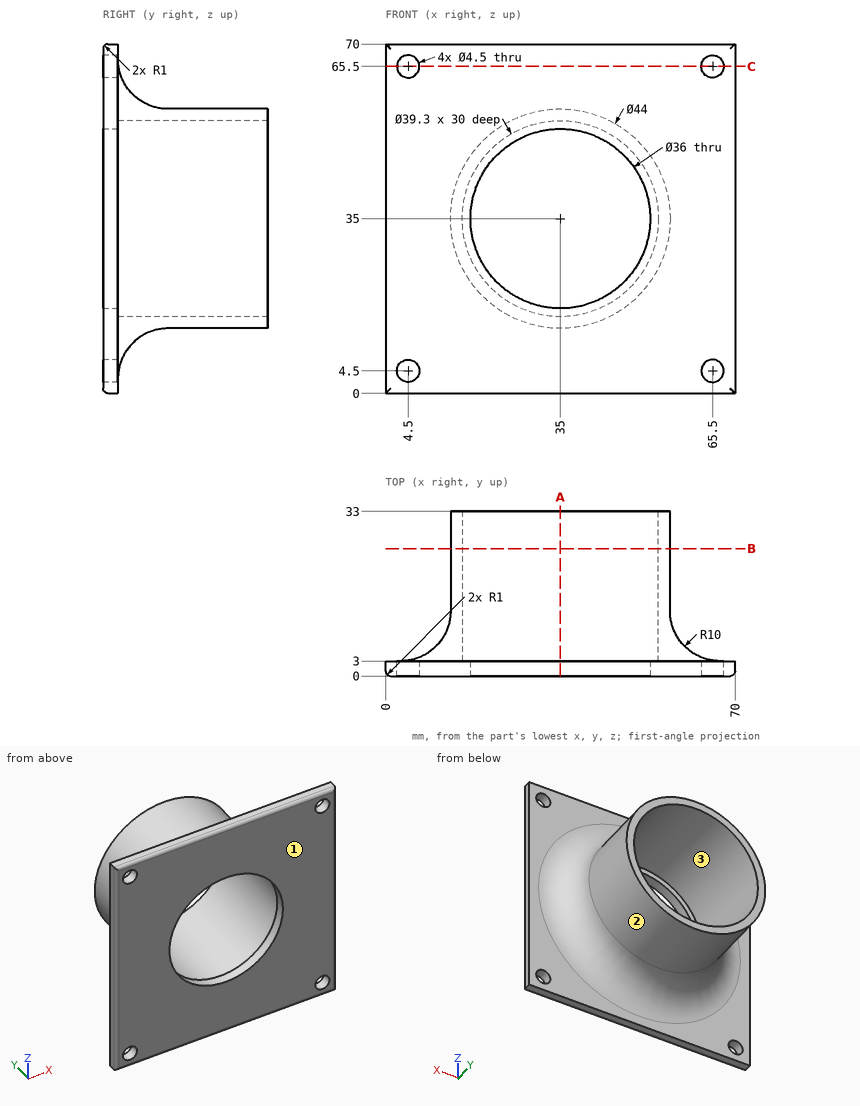
Geometry: see drawing. Coordinates: mm, zero at the bounding-box minimum. Give positions to 0.01 mm unless a question says otherwise; leave off trailing zeros. Order: outer loops, then holes, each group sorted by start corner. A loop starts at its lowest first (then second) coordinate and runs counter-clockwise, first axis right, second up. Notation, with made-up numbers: (67, 3.5) - (93, 3.5) arc R4 ccw to (93, 9.5) - close; hole circle Ø8 at (19, 20.5). An arc over 180 degrees is marked (long way). Use a Markdown table: item, result.
(1) Draft query along Z for the marked faces 1, 2 and 3. Return one class per face: released by +Z, released by -Z, zero draft, split by the parting line, or undercut.
Computed values:
| item | result |
|---|---|
| face 1 | zero draft |
| face 2 | split by the parting line |
| face 3 | undercut |
(2) Section query A-A (x = 35). Output: boundary loops of the cut face in (y, z), then the cut area to 3 significant figures.
Computed values:
| item | result |
|---|---|
| outline | (0, 1) arc R1 ccw to (1, 0) - (3, 0) - (3, 3) arc R10 cw to (13, 13) - (33, 13) - (33, 15.35) - (3, 15.35) - (3, 17) - (0, 17) - close; (0, 53) - (3, 53) - (3, 54.65) - (33, 54.65) - (33, 57) - (13, 57) arc R10 cw to (3, 67) - (3, 70) - (1, 70) arc R1 ccw to (0, 69) - close |
| area | 285 mm2 |
(3) Section query B-B (y = 25.5). Output: boundary loops of the cut face in (x, z).
Computed values:
| item | result |
|---|---|
| outline | circle Ø44 at (35, 35); hole circle Ø39.3 at (35, 35) |
(4) Line query: line 1 (X direction, y = 1.15, z = 65.5); line 2 (Z direction, x = 65.5, y = 0.8); line 3 (X direction, y = 17, z = 35). Output: solid intervals per line, ascending. Write a range as from..to.
Computed values:
| item | result |
|---|---|
| line 1 | x = 0..2.25, 6.75..63.25, 67.75..70 |
| line 2 | z = 0.02..2.25, 6.75..63.25, 67.75..69.98 |
| line 3 | x = 13..15.35, 54.65..57 |
(5) Section query C-C (z = 65.5). State how many separate pieces and enclosed holes the cut face has, then the cut area to 3 significant figures.
Computed values:
| item | result |
|---|---|
| separate pieces | 3 |
| enclosed holes | 0 |
| area | 184 mm2 |
(6) Pin query (flat end, axial travel): pin 1 (2 mm diameter, centred on y = 19, z = 28.5, fed in from +X); pin 2 (8 mm diameter, centred on x = 37, y = 23.5, fed in from -Z); pin 3 (12 mm diameter, centred on y = 20, z = 46, fed in from +X). Return the tip coordinate at first contact, or that it passes through.
Computed values:
| item | result |
|---|---|
| pin 1 | stops at x = 56.3 |
| pin 2 | stops at z = 13 |
| pin 3 | stops at x = 56.42 |
